from build123d import *

# Parameters (mm, degrees)
F0_W     = 0.4
F0_H     = 2.066987
F0_W_2   = 6.166988
F0_H_2   = 0.433013
F0_W_3   = 0.433012
F4_DEPTH = 8


with BuildPart() as f1:
    # F0 (on Front) → F1 (revolve)
    with BuildSketch(Plane.XZ):
        Polygon((-25.239477, -88.669804), (-20.739477, -88.669804), (-20.739477, -83.669804), (-90.739477, -83.669804), (-90.739477, -91.669804), (-37.659028, -91.669804), (-36.239477, -89.21107), (-33.239477, -89.21107), (-33.239477, -87.796821), (-25.239477, -87.796821), align=None)
        Polygon((-26.1410899297, -88.669804), (-25.239477, -88.669804), (-25.239477, -87.796821), align=None)
        Polygon((-32.239477, -88.669804), (-26.1410899297, -88.669804), (-25.239477, -87.796821), (-33.239477, -87.796821), (-32.3025853972, -88.7039624297), align=None)
        Polygon((-33.239477, -87.796821), (-33.239477, -89.21107), (-32.3025853972, -88.7039624297), align=None)
        Polygon((-20.739477, -88.669804), (-20.239477, -88.669804), (-20.239477, -84.169804), (-20.739477, -83.669804), align=None)
        Polygon((-90.739477, -91.669804), (-90.739477, -83.669804), (-91.239477, -84.169804), (-91.239477, -87.049804), (-91.239477, -89.169804), (-91.239477, -89.602817), (-91.239477, -91.669804), align=None)
        with Locations((-91.439477, -90.6363105)):
            Rectangle(F0_W, F0_H)
        with BuildLine():
            Line((-91.639477, -89.602817), (-91.239477, -89.602817))
            Line((-91.239477, -89.602817), (-91.239477, -89.169804))
            ThreePointArc((-91.239477, -89.169804), (-91.439477, -89.369804), (-91.639477, -89.169804))
            Line((-91.639477, -89.169804), (-91.639477, -89.602817))
        make_face()
        with Locations((-94.722971, -89.3863105)):
            Rectangle(F0_W_2, F0_H_2)
        with Locations((-94.722971, -90.6363105)):
            Rectangle(F0_W_2, F0_H)
        with Locations((-98.022971, -90.6363105)):
            Rectangle(F0_W_3, F0_H)
        Polygon((-98.239477, -89.602817), (-97.806465, -89.602817), (-97.806465, -89.169804), align=None)
    revolve(axis=Axis((-57.779478, 0, -91.669804), (-1, 0, 0)))

    # F3 (on offset) → F4 (cut)
    with BuildSketch(Plane.YZ.offset(-33.239477)):
        Polygon((-7, -105.1077917218), (-7, -81.2891572714), (-14.8517033085, -81.2891572714), (-15.7914049923, -106.496937573), align=None)
        Polygon((14.2944240943, -81.2891572714), (7, -81.2891572714), (7, -105.1077917218), (14.2944240943, -107.9208105803), align=None)
    extrude(amount=F4_DEPTH, mode=Mode.SUBTRACT)


solid = f1.part
The model under review builds one solid part; all positions refer to its coordinate system, in mm. A direction names the side the tool comes from. Round coordinates to 2 decimals unless told otherwise and drop trailing zeros. Write each loop counter-clockwise with the first axis right and the second up, starting at its lowest first coordinate (ties: lowest second). Pieces come first, ordered by that corner, then holes. Notation, with made-up numbers: M -32,35 L -21,35 A31 ccw -21,63 Z; hole C 69.25,16 d10. An arc over 180 degrees is marked long. Answer as CSV lines item,"result". Start each with the question number.
Q1. The part is to be moulded in two halves that separate along Z. For faces 1 (the face through (-29, 7, -92)), 2 (the face through (-56.229, 7.932, -92.711)), 3 (the face through (-26.155, 0.132, -94.667)), say which applies: +Z half, -Z half, draft (parallel to the pull), parting line (faces both ways), or undercut.
Q2. Wall thickness on line 1 along X through (y, z) = (3, -92.5); line 2 along Y through (x, z) = (-25, -93.5); line 3 along Z through (x, y) = (-80.5, -3.25): over which ranges is each line inside the solid? List them lowest first.
Q3. Tool access review of faces 4 (the face through (-91.239, 0, -88)), 5 (the face through (-98.239, 0, -92)), 6 (the face through (-29, -7, -92)), 7 (the face through (-34.718, 0.108, -94.126)): name each direction out of +Z, -Z, +X, -X, +Y, -Y from which nothing blocks a thin tool from reaching the whole face with its end or side.
Q4. Clearance check with flat-ended pins moving along their axes: P1, Ø4, axis at x = -36.5, y = 3, coming from the -Z side; P2, Ø8, axis at x = -41.5, z = -86, coming from the -Y side; P3, Ø0.8, axis at y = 7.5, z = -92.5, coming from the -X side. State where each tip first meets the part, or that it passes through.
Q5. Consider section A-A, the plane x = -40. Give the boundary of the cut face in (y, z), then the cut area to 3 significant figures.
Result set:
1,face 1,"draft"
1,face 2,"parting line"
1,face 3,"undercut"
2,line 1,"x = -91.24 to -20.24"
2,line 2,"y = -7.79 to -2.38, 2.38 to 7.79"
2,line 3,"z = -98.98 to -84.36"
3,face 4,"-X"
3,face 5,"+Z, -Z, -X, +Y, -Y"
3,face 6,"+Z, -Z, -Y"
3,face 7,"+X"
4,P1,"stops at z = -99.61"
4,P2,"stops at y = -7.82"
4,P3,"stops at x = -91.24"
5,outline,"C 0,-91.67 d16"
5,area,"201 mm²"
